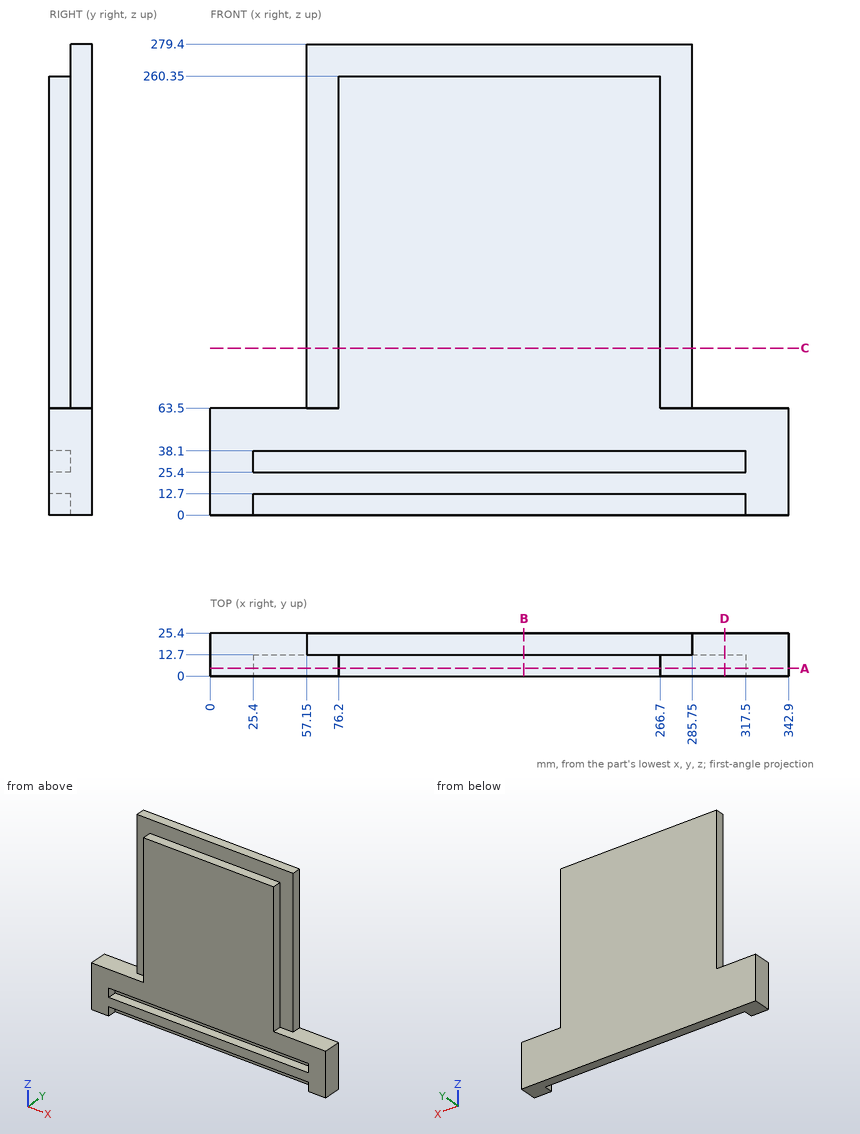
Can you work these out from the drawing? Everything is in mm from the part's minimum corner. Coordinates: 2 decimals unless noted, no trailing zeros. Order: outer loops, then holes, each group sorted by start corner. A loop starts at its lowest first (then second) coordinate and runs counter-clockwise, first axis right, second up. Notation, with made-up numbers: M 14,58 L 69,58 A9 ccw 69,70 Z; hole C 65,14.25 d3. An arc over 180 degrees is marked long. Answer as CSV lines item,"result". Start each with the question number.
1. I need wall thicknesses on line 1 (Z direction, x = 186.5, y = 5.75); line 2 (X direction, y = 12.25, z = 211.5); line 3 (X direction, y = 14.75, z = 107). Which ranges of each line are inside material? Lowest first, please. Write a range as [from, to].
2. I want a section at B-B, the plane x = 186. Write out the boundary of the cut face in (y, z), and give its area (3 significant figures).
3. I want a section at D-D, the plane x = 305. Write out the boundary of the cut face in (y, z).
4. For pin 1 (6.5 mm diameter, centred on y = 7.5, z = 207.5, fed in from +X); pin 2 (14 mm diameter, centred on x = 204.5, y = 5.5, fed in from +Z); pin 3 (10 mm diameter, centred on x = 171, y = 7.5, fed in from -Z), each with a flat end and sliding along its axis, tell me the tip position at first contact or that it passes through.
5. I want a section at C-C, the plane z = 99. Write out the boundary of the cut face in (x, y), and give its area (3 significant figures).
6. I want a section at A-A, the plane y = 4.5. Write out the boundary of the cut face in (x, z), and give its area (3 significant figures).
Recorded:
1,line 1,"z = [12.7, 25.4], [38.1, 260.35]"
1,line 2,"x = [76.2, 266.7]"
1,line 3,"x = [57.15, 285.75]"
2,outline,"M 0,12.7 L 12.7,12.7 L 12.7,0 L 25.4,0 L 25.4,279.4 L 12.7,279.4 L 12.7,260.35 L 0,260.35 L 0,38.1 L 12.7,38.1 L 12.7,25.4 L 0,25.4 Z"
2,area,"6,530 mm2"
3,outline,"M 0,12.7 L 12.7,12.7 L 12.7,0 L 25.4,0 L 25.4,63.5 L 0,63.5 L 0,38.1 L 12.7,38.1 L 12.7,25.4 L 0,25.4 Z"
4,pin 1,"stops at x = 266.7"
4,pin 2,"stops at z = 260.35"
4,pin 3,"stops at z = 12.7"
5,outline,"M 57.15,12.7 L 76.2,12.7 L 76.2,0 L 266.7,0 L 266.7,12.7 L 285.75,12.7 L 285.75,25.4 L 57.15,25.4 Z"
5,area,"5,320 mm2"
6,outline,"M 0,0 L 25.4,0 L 25.4,12.7 L 317.5,12.7 L 317.5,0 L 342.9,0 L 342.9,63.5 L 266.7,63.5 L 266.7,260.35 L 76.2,260.35 L 76.2,63.5 L 0,63.5 Z; hole M 25.4,25.4 L 317.5,25.4 L 317.5,38.1 L 25.4,38.1 Z"
6,area,"51,900 mm2"
